```python
from build123d import *

# Parameters (mm, degrees)
ESBO_O1_R                = 1.5
RESSALTO_EXTRUS_O1_DEPTH = 0.25
RESSALTO_EXTRUS_O2_START = 0.25
ESBO_O1_3_R              = 0.75
RESSALTO_EXTRUS_O2_DEPTH = 0.1
CORTE_EXTRUS_O1_START    = -0.25
ESBO_O1_4_R              = 0.75
CORTE_EXTRUS_O1_DEPTH    = 0.1
FILETE1_R                = 2


with BuildPart() as part:
    # Esboço1 → Ressalto-extrusão1 (new, symmetric)
    with BuildSketch(Plane(origin=(0, 0, 0), x_dir=(1, 0, 0), z_dir=(0, 1, 0))):
        with BuildLine():
            Line((-14.269532703, -20.99999997), (14.269532672, -20.99999997))
            ThreePointArc((14.269532672, -20.99999997), (17.748380193, -17.748380193), (20.99999997, -14.269532672))
            Line((20.99999997, -14.269532672), (20.99999997, -0.699999985))
            Line((20.99999997, -0.699999985), (20.49999997, -0.699999985))
            Line((20.49999997, -0.699999985), (20.49999997, 0.700000015))
            Line((20.49999997, 0.700000015), (20.99999997, 0.700000015))
            Line((20.99999997, 0.700000015), (20.99999997, 14.269532702))
            ThreePointArc((20.99999997, 14.269532702), (17.748380193, 17.748380223), (14.269532672, 21))
            Line((14.269532672, 21), (-14.269532702, 21))
            ThreePointArc((-14.269532702, 21), (-17.748380223, 17.748380223), (-21, 14.269532703))
            Line((-21, 14.269532703), (-21, -14.269532672))
            ThreePointArc((-21, -14.269532672), (-17.748380223, -17.748380193), (-14.269532703, -20.99999997))
        make_face()
        with Locations(Location((15.5, 15.5, 0), (0, 0, 270))):
            Circle(ESBO_O1_R, mode=Mode.SUBTRACT)
        with Locations(Location((-15.5, 15.5, 0), (0, 0, 270))):
            Circle(ESBO_O1_R, mode=Mode.SUBTRACT)
        with Locations(Location((-15.5, -15.5, 0), (0, 0, 270))):
            Circle(ESBO_O1_R, mode=Mode.SUBTRACT)
        with Locations(Location((15.5, -15.5, 0), (0, 0, 270))):
            Circle(ESBO_O1_R, mode=Mode.SUBTRACT)
        Polygon((19.25, 7.973611076), (7.973611076, 19.25), (-7.973611076, 19.25), (-19.25, 7.973611076), (-19.25, -7.973611076), (-7.973611076, -19.25), (7.973611076, -19.25), (19.25, -7.973611076), align=None, mode=Mode.SUBTRACT)
    extrude(amount=RESSALTO_EXTRUS_O1_DEPTH, both=True)

    # Esboço1<3> → Ressalto-extrusão2 (add)
    with BuildSketch(Plane(origin=(0, 0, 0), x_dir=(1, 0, 0), z_dir=(0, 1, 0)).offset(RESSALTO_EXTRUS_O2_START)):
        with Locations(Location((-18.915106397, 11.844038585, 0), (0, 0, 90))):
            Circle(ESBO_O1_3_R)
        with Locations(Location((-11.844038585, 18.915106397, 0), (0, 0, 90))):
            Circle(ESBO_O1_3_R)
        with Locations(Location((11.844038585, 18.915106397, 0), (0, 0, 90))):
            Circle(ESBO_O1_3_R)
        with Locations(Location((18.915106397, 11.844038585, 0), (0, 0, 90))):
            Circle(ESBO_O1_3_R)
        with Locations(Location((18.915106397, -11.844038585, 0), (0, 0, 90))):
            Circle(ESBO_O1_3_R)
        with Locations(Location((11.844038585, -18.915106397, 0), (0, 0, 90))):
            Circle(ESBO_O1_3_R)
        with Locations(Location((-11.844038585, -18.915106397, 0), (0, 0, 90))):
            Circle(ESBO_O1_3_R)
        with Locations(Location((-18.915106397, -11.844038585, 0), (0, 0, 90))):
            Circle(ESBO_O1_3_R)
    extrude(amount=RESSALTO_EXTRUS_O2_DEPTH)

    # Esboço1<4> → Corte-extrusão1 (cut)
    with BuildSketch(Plane(origin=(0, 0, 0), x_dir=(1, 0, 0), z_dir=(0, 1, 0)).offset(CORTE_EXTRUS_O1_START)):
        with Locations(Location((-11.844038585, -18.915106397, 0), (0, 0, 90))):
            Circle(ESBO_O1_4_R)
        with Locations(Location((18.915106397, -11.844038585, 0), (0, 0, 90))):
            Circle(ESBO_O1_4_R)
        with Locations(Location((-18.915106397, 11.844038585, 0), (0, 0, 90))):
            Circle(ESBO_O1_4_R)
        with Locations(Location((-18.915106397, -11.844038585, 0), (0, 0, 90))):
            Circle(ESBO_O1_4_R)
        with Locations(Location((11.844038585, -18.915106397, 0), (0, 0, 90))):
            Circle(ESBO_O1_4_R)
        with Locations(Location((18.915106397, 11.844038585, 0), (0, 0, 90))):
            Circle(ESBO_O1_4_R)
        with Locations(Location((11.844038585, 18.915106397, 0), (0, 0, 90))):
            Circle(ESBO_O1_4_R)
        with Locations(Location((-11.844038585, 18.915106397, 0), (0, 0, 90))):
            Circle(ESBO_O1_4_R)
    extrude(amount=CORTE_EXTRUS_O1_DEPTH, mode=Mode.SUBTRACT)

    # Filete1
    filete1_edges = [part.edges().sort_by_distance(p)[0] for p in [
        (-14.269532703, 0, 20.99999997),
        (14.269532672, 0, 20.99999997),
        (20.99999997, 0, 14.269532672),
        (20.99999997, 0, -14.269532702),
        (14.269532672, 0, -21),
        (-14.269532702, 0, -21),
        (-21, 0, -14.269532703),
        (-21, 0, 14.269532672),
    ]]
    fillet(filete1_edges, radius=FILETE1_R)


solid = part.part
```
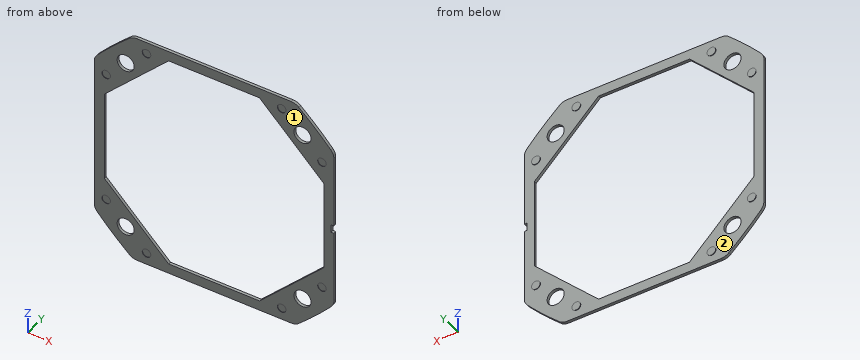
Verification items for the finished model (mm, model axes). Face numbers are marked on the shaded views. A direction names the side the tool comes from. Coordinates: 2 decimals unless noted, no trailing zeros. Write each loop counter-clockwise with the first axis right and the second up, starting at its lowest first coordinate (ties: lowest second). Pieces come first, ordered by that corner, then holes. Notation, with made-up numbers: (-40, 37) - (4, 37) arc R20 cw to (4, 57) - close; hole circle Ø9 at (19.5, 27). An arc over 180 degrees is marked (long way). One line per question, with ' | ' between items. Start each with the question number.
1. Section check B-B (x = 5). Enter the section's corners in (y, z), plus the area to 3 significant figures.
2. Access from +Z, -Z, +X, -X, +Y, -Y to the whole of each face (thin tool, end or side, straight path). Record for the marked faces 1 and 2.
3. Section check D-D (z = -15.5). Enter the section's corners in (x, y), plus the area to 3 significant figures.
4. Gauge pin test, flat ends, axial feed: P1, Ø1.8, axis at x = 15.5, z = 15.5, coming from the -Y side; P2, Ø4, axis at x = 15.5, z = -15.5, coming from the +Y side. Record the tip position at first contact, or that the pin passes through.
5. Section check C-C (y = -0.05). Count the separate pieces of the cut face and the enclosed holes in it, plus the area to 3 significant figures.
6. Section check A-A (z = 1.5). Enter the section's corners in (x, y), plus the area to 3 significant figures.
7. Material ranges on line 1 along X through (y, z) = (0.15, 2); line 2 along X through (y, z) = (-0.2, 15), recorded low to high.
Computed values:
1) outline: (-0.25, -21) - (0.25, -21) - (0.25, -19.25) - (-0.25, -19.25) - close; (-0.25, 19.25) - (0.25, 19.25) - (0.25, 21) - (-0.25, 21) - close | area: 1.75 mm²
2) face 1: +Z, -Z, +X, -X, -Y | face 2: +Y
3) outline: (-19.9, -0.25) - (-17, -0.25) - (-17, 0.25) - (-19.9, 0.25) - close; (-14, -0.25) - (-11.72, -0.25) - (-11.72, 0.25) - (-14, 0.25) - close; (11.72, -0.25) - (14, -0.25) - (14, 0.25) - (11.72, 0.25) - close; (17, -0.25) - (19.9, -0.25) - (19.9, 0.25) - (17, 0.25) - close | area: 5.18 mm²
4) P1: through | P2: y = 0.25
5) separate pieces: 1 | enclosed holes: 5 | area: 420 mm²
6) outline: (-21, -0.25) - (-19.25, -0.25) - (-19.25, 0.25) - (-21, 0.25) - close; (19.25, -0.25) - (21, -0.25) - (21, 0.25) - (19.25, 0.25) - close | area: 1.75 mm²
7) line 1: -21 to -19.25, 19.25 to 21 | line 2: -20.35 to -16.91, -14.09 to -12.22, 12.22 to 14.09, 16.91 to 20.35
